Geometry check sheet. Reference: the model listing, model coordinates, mm. A direction names the side the tool comes from. Give positions to 0.01 mm unless a question says otherwise; leave off trailing zeros. Loops run counter-clockwise (first coordinate to the right, second up) from the corner with the lowest first, then second, coordinate; pieces in that order, holes last. Notation, with made-up numbers: (-29.75, 65) -> (5.25, 65) arc R20 cw to (5.25, 69) -> close; hole circle Ø1 at (24.5, -12.5). An arc over 180 degrees is marked (long way). Answer as a JSON object with one key per item and string values.
Autodesk Inventor part; units mm, degrees
ref_plane "YZ Plane" through (0, 0, 0) normal (1, 0, 0) x (0, 1, 0)
ref_plane "XZ Plane" through (0, 0, 0) normal (0, 1, 0) x (-1, 0, 0)
ref_plane "XY Plane" through (0, 0, 0) normal (0, 0, 1) x (1, 0, 0)
ref_plane "Work Plane1" through (0, 0, 0) normal (0, 0, 1) x (1, 0, 0)
sketch "Sketch1" plane through (0, 0, 0) normal (0, 0, 1) x (1, 0, 0)
  circle A0 centre (-25.4098, 20.8167) radius 8
  circle A1 centre (-109.1654, 20.8167) radius 8
  circle A2 centre (-67.2876, 20.8167) radius 11.5
  line L0 (-56.2876, 67.31) -> (-56.2876, 59.315)
  line L1 (-56.2876, 59.315) -> (-61.2876, 59.315)
  line L2 (-61.2876, 59.315) -> (-56.2876, 54.315)
  line L3 (-56.2876, 54.315) -> (-56.2876, 45.32)
  line L4 (-56.2876, 45.32) -> (-64.2876, 45.32)
  line L5 (-64.2876, 51.32) -> (-64.2876, 45.32)
  line L6 (-70.2876, 51.32) -> (-64.2876, 51.32)
  line L7 (-70.2876, 45.32) -> (-70.2876, 51.32)
  line L8 (-70.2876, 45.32) -> (-78.2876, 45.32)
  line L9 (-78.2876, 45.32) -> (-78.2876, 54.315)
  line L10 (-78.2876, 54.315) -> (-73.2876, 59.315)
  line L11 (-73.2876, 59.315) -> (-78.2876, 59.315)
  line L12 (-78.2876, 59.315) -> (-78.2876, 67.31)
  line L13 (-78.2876, 67.31) -> (-105.9385, 67.31)
  line L14 (-105.9385, 67.31) -> (-141.1337, 6.35)
  line L15 (-141.1337, 6.35) -> (-9.2697, 6.35)
  line L16 (-9.2697, 6.35) -> (-9.2697, 67.31)
  line L17 (-9.2697, 67.31) -> (-56.2876, 67.31)
  circle A3 centre (-109.1654, 20.8167) radius 8
  circle A4 centre (-25.4098, 20.8167) radius 8
  circle A5 centre (-67.2876, 20.8167) radius 11.5
  line L18 (-77.2876, 46.815) -> (-57.2876, 46.815)
  line L19 (-57.2876, 46.815) -> (-57.2876, 66.815)
  line L20 (-57.2876, 66.815) -> (-77.2876, 66.815)
  line L21 (-77.2876, 66.815) -> (-77.2876, 46.815)
  line L22 (-77.2876, 46.815) -> (-57.2876, 66.815) construction
  line L23 (-57.2876, 46.815) -> (-77.2876, 66.815) construction
  line L24 (-79.9876, 69.515) -> (-54.5876, 69.515)
  line L25 (-54.5876, 69.515) -> (-54.5876, 44.115)
  line L26 (-54.5876, 44.115) -> (-79.9876, 44.115)
  line L27 (-79.9876, 44.115) -> (-79.9876, 69.515)
  line L28 (-79.9876, 69.515) -> (-54.5876, 44.115) construction
  line L29 (-54.5876, 69.515) -> (-79.9876, 44.115) construction
  point P0 (0, 0)
  point P1 (-67.2876, 56.815)
  dimension "d0" = 20
  dimension "d1" = 20
  dimension "d2" = 25.4
  dimension "d3" = 25.4
extrude "Extrusion1" add sketch "Sketch1" along normal blind 25.4 contours L17 L25 L26 L27 L13 L12 L11 L21 L10 L9 L8 L7 L18 L5 L4 L3 L2 L19 L1 L0 | L0 L1 L19 L20 L21 L11 L12 L13 L27 L24 L25 L17 | L2 L3 L4 L5 L18 L19 | L7 L8 L9 L10 L21 L18
sketch "Sketch2" plane through (0, 0, 25.4) normal (0, 0, 1) x (1, 0, 0)
  line L0 (-56.2876, 67.31) -> (-56.2876, 59.315)
  line L1 (-56.2876, 59.315) -> (-61.2876, 59.315)
  line L2 (-61.2876, 59.315) -> (-56.2876, 54.315)
  line L3 (-56.2876, 54.315) -> (-56.2876, 45.32)
  line L4 (-56.2876, 45.32) -> (-64.2876, 45.32)
  line L5 (-64.2876, 51.32) -> (-64.2876, 45.32)
  line L6 (-70.2876, 51.32) -> (-64.2876, 51.32)
  line L7 (-70.2876, 45.32) -> (-70.2876, 51.32)
  line L8 (-70.2876, 45.32) -> (-78.2876, 45.32)
  line L9 (-78.2876, 45.32) -> (-78.2876, 54.315)
  line L10 (-78.2876, 54.315) -> (-73.2876, 59.315)
  line L11 (-73.2876, 59.315) -> (-78.2876, 59.315)
  line L12 (-78.2876, 59.315) -> (-78.2876, 67.31)
  line L13 (-78.2876, 67.31) -> (-105.9385, 67.31)
  line L14 (-105.9385, 67.31) -> (-141.1337, 6.35)
  line L15 (-141.1337, 6.35) -> (-9.2697, 6.35)
  line L16 (-9.2697, 6.35) -> (-9.2697, 67.31)
  line L17 (-9.2697, 67.31) -> (-56.2876, 67.31)
  circle A0 centre (-109.1654, 20.8167) radius 8
  circle A1 centre (-25.4098, 20.8167) radius 8
  circle A2 centre (-67.2876, 20.8167) radius 11.5
  circle A3 centre (-25.4098, 20.8167) radius 4
  point P0 (0, 0)
  dimension "d6" = 8
properties part number "Right X End"
1) Section check B-B on z = 22.25. Record the cut outline in (x, y) (3 decimals).
Geometry check:
{"outline": "(-79.988, 44.115) -> (-54.588, 44.115) -> (-54.588, 69.515) -> (-79.988, 69.515) -> close; hole (-77.288, 46.815) -> (-57.288, 46.815) -> (-57.288, 66.815) -> (-77.288, 66.815) -> close"}
2) Section check A-A on y = 51.75. Record the cut outline in (x, z).
Geometry check:
{"outline": "(-79.99, 0) -> (-77.29, 0) -> (-77.29, 25.4) -> (-79.99, 25.4) -> close; (-57.29, 0) -> (-54.59, 0) -> (-54.59, 25.4) -> (-57.29, 25.4) -> close"}
3) Draft check along X on faces 3 (the face through (-54.588, 57, 13)), 4 (the face through (-67, 66.815, 13)), 5 (the face through (-67, 44.115, 13)). Enter one of: pulls with the +X half, pulls with the -X half, needs draft (parallel to the pull), parting line crosses it, or undercut.
Geometry check:
{"face 3": "pulls with the +X half", "face 4": "undercut", "face 5": "needs draft"}
4) Tool access check on faces 1 (the face through (-57.288, 57, 13)), 2 (the face through (-67, 69.515, 13)). Record the directions out of +Z, -Z, +X, -X, +Y, -Y that give a thin tool (end or side, any length) a straight path to the whole face; none if there is none.
Geometry check:
{"face 1": "+Z, -Z", "face 2": "+Z, -Z, +X, -X, +Y"}
5) Section check C-C on x = -75.5. Record the cut outline in (y, z) (3 decimals), plus the area to 3 significant figures.
Geometry check:
{"outline": "(44.115, 0) -> (46.815, 0) -> (46.815, 25.4) -> (44.115, 25.4) -> close; (66.815, 0) -> (69.515, 0) -> (69.515, 25.4) -> (66.815, 25.4) -> close", "area": "137 mm2"}
6) Material ranges on line 1 along X through (y, z) = (53.5, 10.25); line 2 along Y through (x, z) = (-74.75, 13.25) (3 decimals), recorded low to high. Write a range as from..to.
Geometry check:
{"line 1": "x = -79.99..-77.29, -57.29..-54.59", "line 2": "y = 44.115..46.815, 66.815..69.515"}
